Design review of the part built by this model. Coordinates are the model's own, in mm. A direction names the side the tool comes from. Round coordinates to 2 decimals unless told otherwise and drop trailing zeros. Order: outer loops, then holes, each group sorted by start corner. A loop starts at its lowest first (then second) coordinate and runs counter-clockwise, first axis right, second up. Notation, with made-up numbers: M 53,82 L 87,82 A12 ccw 87,89 Z; hole C -29,9.5 d3. An arc over 180 degrees is marked long. Write item = value, one per line. Start each with the question number.
```python
from build123d import *

# Parameters (mm, degrees)
PIN_START            = 13
PIN_BOSS_FRONT_DEPTH = 31.5
PIN_START_2          = -44.5
PIN_BOSS_REAR_DEPTH  = 31.5
PIN_BORE_DEPTH       = 78.481739955
PIN_BORE_DEPTH_BACK  = 78.481739955
SKETCH4_R            = 11.85
SKETCH5_W            = 4.1
SKETCH5_H            = 1.5
SKETCH5_H_2          = 3
SKETCH6_R            = 17
SKETCH6_R_2          = 15
VALVE_RELIEFS_DEPTH  = 1.5


with BuildPart() as part:
    # Sketch1 → Piston Body (revolve)
    with BuildSketch(Plane.XY, mode=Mode.PRIVATE) as piston_body_sk:
        with BuildLine():
            Line((0, 33.8), (48.1, 33.8))
            ThreePointArc((48.1, 33.8), (48.948528137, 33.448528137), (49.3, 32.6))
            Line((49.3, 32.6), (49.3, -26))
            Line((49.3, -26), (44.3, -26))
            Line((44.3, -26), (44.3, 19))
            Line((44.3, 19), (0, 19))
            Line((0, 19), (0, 33.8))
        make_face()
    revolve(piston_body_sk.sketch.rotate(Axis((0, -60, 0), (0, 1, 0)), 90), axis=Axis((0, -60, 0), (0, 1, 0)))

    # Sketch2 → Pin Boss Front (add)
    with BuildSketch(Plane.XY.offset(PIN_START)):
        with BuildLine():
            Line((-17, 19.5), (-17, -1.7))
            ThreePointArc((-17, -1.7), (-12.518733752, -12.518733752), (-1.7, -17))
            Line((-1.7, -17), (1.7, -17))
            ThreePointArc((1.7, -17), (12.518733752, -12.518733752), (17, -1.7))
            Line((17, -1.7), (17, 19.5))
            Line((17, 19.5), (-17, 19.5))
        make_face()
    extrude(amount=PIN_BOSS_FRONT_DEPTH)

    # Sketch3 → Pin Boss Rear (add)
    with BuildSketch(Plane.XY.offset(PIN_START_2)):
        with BuildLine():
            Line((-17, 19.5), (-17, -1.7))
            ThreePointArc((-17, -1.7), (-12.518733752, -12.518733752), (-1.7, -17))
            Line((-1.7, -17), (1.7, -17))
            ThreePointArc((1.7, -17), (12.518733752, -12.518733752), (17, -1.7))
            Line((17, -1.7), (17, 19.5))
            Line((17, 19.5), (-17, 19.5))
        make_face()
    extrude(amount=PIN_BOSS_REAR_DEPTH)

    # Sketch4 → Pin Bore (cut, two sides: drawn at the far end of the back side and taken through both)
    with BuildSketch(Plane.XY.offset(-PIN_BORE_DEPTH_BACK)):
        Circle(SKETCH4_R)
    extrude(amount=PIN_BORE_DEPTH + PIN_BORE_DEPTH_BACK, mode=Mode.SUBTRACT)

    # Sketch5 → Ring Grooves (revolve, cut)
    with BuildSketch(Plane.XY, mode=Mode.PRIVATE) as ring_grooves_sk:
        with Locations((48.45, 27.75)):
            Rectangle(SKETCH5_W, SKETCH5_H)
        with Locations((48.45, 23.25)):
            Rectangle(SKETCH5_W, SKETCH5_H)
        with Locations((48.45, 18)):
            Rectangle(SKETCH5_W, SKETCH5_H_2)
    revolve(ring_grooves_sk.sketch.rotate(Axis((0, -60, 0), (0, 1, 0)), 90), axis=Axis((0, -60, 0), (0, 1, 0)), mode=Mode.SUBTRACT)

    # Sketch6 → Valve Reliefs (cut)
    with BuildSketch(Plane(origin=(0, 33.8, 0), x_dir=(1, 0, 0), z_dir=(0, 1, 0))):
        with Locations(Location((-20, 12, 0), (0, 0, 270))):
            Circle(SKETCH6_R)
        with Locations(Location((20, -12, 0), (0, 0, 270))):
            Circle(SKETCH6_R_2)
    extrude(amount=-VALVE_RELIEFS_DEPTH, mode=Mode.SUBTRACT)


solid = part.part
```
(1) Consider section C-C, the plane x = -9.5. State how many separate pieces and enclosed holes the cut face has, then the cut area to 3 significant figures.
(2) For faces 1 (the face through (-20, 32.3, -12)), 2 (the face through (-33, 19.5, 33)), 3 (the face through (-12.637, -12.399, -28.853)), 4 (the face through (18.88, -5.05, -45.54)), list the 3-axis set-ups (+Z, -Z, +X, -X, +Y, -Y) from which the entire face can be reached by the end or side of a thin tool; tool diameter is ignored.
(3) Draft analysis for pull direction X (two halves, no side actions). For faces 5 (the face through (-33, 22.5, 33)), 6 (the face through (20, 32.3, 12)), 7 (the face through (-31.36, 23.26, 34.2)), state which applies: pulls with the +X half, pulls with the -X half, needs draft (parallel to the pull), parting line crosses it, or undercut.
(4) Insertion check: pin 1 (6 mm diameter, centred on y = 8.5, z = 22, fed in from -X); pin 2 (1 mm diameter, centred on y = -8, z = -4, fed in from +X); pin 3 (23 mm diameter, centred on y = 7.5, z = -27, fed in from -X); pin 4 (5 mm diameter, centred on x = -6, y = 7, fed in from -Z). Each pin has a flat end and moves straight along its axis. Give the tip position at first contact, or say it passes through.
(5) For line 1 along Y through (x, z) = (-44, 19.5); line 2 along Y through (x, z) = (0, -32); line 3 along X through (y, z) = (-5.5, -30), list the stretches that pass through material, from the lowest coordinate up. Write a range as [from, to].
(6) Consider section B-B, the plane y = 10.5. Write out the cut boundary in (x, z), then the cut area to 3 significant figures.
(7) Consider section A-A, the plane y = 0. Write out the cut boundary in (x, z), then the cut area to 3 significant figures.
Completed:
q1.separate_pieces = 3
q1.enclosed_holes = 0
q1.area = 2,860 mm2
q2.face_1 = +Y
q2.face_2 = none
q2.face_3 = -Y
q2.face_4 = +Y, -Y
q3.face_5 = needs draft
q3.face_6 = undercut
q3.face_7 = parting line crosses it
q4.pin_1 = -45.49
q4.pin_2 = 49.18
q4.pin_3 = -46.8
q4.pin_4 = through
q5.line_1 = [-26, 16.5], [19.5, 22.5], [24, 27], [28.5, 33.8]
q5.line_2 = [-17, -11.85], [11.85, 33.8]
q5.line_3 = [-39.12, -32.6], [-16.52, -10.5], [10.5, 16.52], [32.6, 39.12]
q6.outline = M -17,-40.91 A44.3 cw -17,40.91 L -17,13 L -5.49,13 L -5.49,48.99 A49.3 ccw -5.49,-48.99 L -5.49,-13 L -17,-13 Z; M 5.49,-48.99 A49.3 ccw 5.49,48.99 L 5.49,13 L 17,13 L 17,40.91 A44.3 cw 17,-40.91 L 17,-13 L 5.49,-13 Z
q6.area = 2,730 mm2
q7.outline = M -17,-40.91 A44.3 cw -17,40.91 L -17,13 L -11.85,13 L -11.85,47.85 A49.3 ccw -11.85,-47.85 L -11.85,-13 L -17,-13 Z; M 11.85,-47.85 A49.3 ccw 11.85,47.85 L 11.85,13 L 17,13 L 17,40.91 A44.3 cw 17,-40.91 L 17,-13 L 11.85,-13 Z
q7.area = 1,830 mm2
